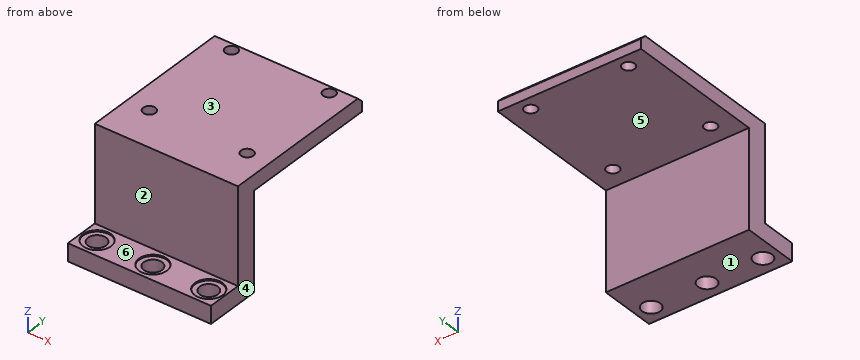
from build123d import *

# Parameters (mm, degrees)
EXTRUDE_1_DEPTH                 = 205
HOLE_WIZARD_M20_1_D             = 17.5
PATTERN_LINEAR_1_COUNT          = 2
PATTERN_LINEAR_1_PITCH          = 140
PATTERN_LINEAR_1_COUNT_DIR2     = 2
PATTERN_LINEAR_1_PITCH_DIR2     = 152
HOLE_WIZARD_M20_1_2_D           = 26
HOLE_WIZARD_M20_1_2_CBORE_D     = 40
HOLE_WIZARD_M20_1_2_CBORE_DEPTH = 2
PATTERN_LINEAR_2_COUNT          = 3
PATTERN_LINEAR_2_PITCH          = 80
CHAMFER_1_SIZE                  = 8


with BuildPart() as part:
    # 草图1 → 凸台-拉伸1 (new body)
    with BuildSketch(Plane(origin=(0, 0, 0), x_dir=(0, 0, -1), z_dir=(1, 0, 0))):
        Polygon((0, 0), (137, 0), (137, -50), (162, -50), (162, 30), (22, 30), (22, 230), (0, 230), align=None)
    extrude(amount=EXTRUDE_1_DEPTH)

    # Hole Wizard M20 _1 (through all)
    with Locations(Plane(origin=(32.5, 211, 0), x_dir=(1, 0, 0), z_dir=(0, 0, 1))):
        with Locations((0, 0)):
            hole_wizard_m20_1 = Hole(HOLE_WIZARD_M20_1_D / 2)

    # 阵列(线性)1: Hole Wizard M20 _1 2 × 2
    with Locations(*[(i * PATTERN_LINEAR_1_PITCH, -j * PATTERN_LINEAR_1_PITCH_DIR2, 0) for i in range(PATTERN_LINEAR_1_COUNT) for j in range(PATTERN_LINEAR_1_COUNT_DIR2) if (i, j) != (0, 0)]):
        add(hole_wizard_m20_1, mode=Mode.SUBTRACT)

    # Hole Wizard M20 _1 2 (through all)
    with Locations(Plane(origin=(22.5, -25, -137), x_dir=(0, 1, 0), z_dir=(0, 0, 1))):
        with Locations((0, 0)):
            hole_wizard_m20_1_2 = CounterBoreHole(HOLE_WIZARD_M20_1_2_D / 2, HOLE_WIZARD_M20_1_2_CBORE_D / 2, HOLE_WIZARD_M20_1_2_CBORE_DEPTH)

    # 阵列(线性)2: Hole Wizard M20 _1 2 ×3
    with Locations(*[(i * PATTERN_LINEAR_2_PITCH, 0, 0) for i in range(1, PATTERN_LINEAR_2_COUNT)]):
        add(hole_wizard_m20_1_2, mode=Mode.SUBTRACT)

    # 倒角1
    chamfer_1_edges = [part.edges().sort_by_distance(p)[0] for p in [
        (102.5, 230, 0),
    ]]
    chamfer(chamfer_1_edges, length=CHAMFER_1_SIZE)


solid = part.part
Source: CAD feature listing. Evaluate the final solid. Frame: model axes, mm. Face numbers are marked on the shaded views. A direction names the side the tool comes from. Round coordinates to 2 decimals unless told otherwise and drop trailing zeros. Loops run counter-clockwise (first coordinate to the right, second up) from the corner with the lowest first, then second, coordinate; pieces in that order, holes last. Notation, with made-up numbers: (-28, 5) - (-10, 5) arc R23 ccw to (-10, 41) - close; hole circle Ø3 at (-18, 46). An arc over 180 degrees is marked (long way). Write item = value, one per line. Start each with the question number.
Item 1: Section query C-C on x = 155. Output: boundary loops of the cut face in (y, z), plus the area to 3 significant figures.
Item 2: Section query B-B on x = 102.5. Output: boundary loops of the cut face in (y, z), plus the area to 3 significant figures.
Item 3: First-contact query: pin 1 Ø1.5 at (x, z) = (33.5, -42) entering from +Y; pin 2 Ø20 at (x, y) = (106.5, -26) entering from +Z; pin 3 Ø15.5 at (x, y) = (102.5, -25) entering from +Z (3 decimals); pin 4 Ø25 at (x, y) = (69.5, -33) entering from +Z. Flat tips, straight axial feed; report the tip coordinate or a pass-through.
Item 4: Reachability of the marked faces 4, 5 and 6 from +Z, -Z, +X, -X, +Y, -Y: full face, straight path, thin tool, end or side. Return the list, or none.
Item 5: Mould query, pull axis Z, two halves, no side actions, for the marked faces 1, 2 and 3. Classes: released by +Z, released by -Z, zero draft, split by the parting line, or undercut.
Item 6: Section query A-A on y = 211. Output: boundary loops of the cut face in (x, z), plus the area to 3 significant figures.
Item 7: Section query D-D on z = -104. Output: boundary loops of the cut face in (x, y), plus the area to 3 significant figures.
Item 8: Material intervals for line 1 (X direction, y = -25, z = -151); line 2 (X direction, y = -25, z = -137.6); line 3 (Y direction, x = 148.5, z = -101.5), sorted ascending.
Results list:
q1.outline = (-50, -162) - (30, -162) - (30, -22) - (230, -22) - (230, -8) - (222, 0) - (0, 0) - (0, -137) - (-50, -137) - close
q1.area = 10,500 mm²
q2.outline = (-50, -162) - (-38, -162) - (-38, -139) - (-45, -139) - (-45, -137) - (-50, -137) - close; (-12, -162) - (30, -162) - (30, -22) - (230, -22) - (230, -8) - (222, 0) - (0, 0) - (0, -137) - (-5, -137) - (-5, -139) - (-12, -139) - close
q2.area = 9,800 mm²
q3.pin_1 = 30
q3.pin_2 = -139
q3.pin_3 = through
q3.pin_4 = -137
q4.face_4 = +Z, -Z, +X, +Y, -Y
q4.face_5 = -Z, +X, -X, +Y
q4.face_6 = +Z, +X, -X, -Y
q5.face_1 = released by -Z
q5.face_2 = zero draft
q5.face_3 = released by +Z
q6.outline = (0, -22) - (23.75, -22) - (23.75, 0) - (0, 0) - close; (41.25, -22) - (163.75, -22) - (163.75, 0) - (41.25, 0) - close; (181.25, -22) - (205, -22) - (205, 0) - (181.25, 0) - close
q6.area = 3,740 mm²
q7.outline = (0, 0) - (205, 0) - (205, 30) - (0, 30) - close
q7.area = 6,150 mm²
q8.line_1 = 0 to 9.5, 35.5 to 89.5, 115.5 to 169.5, 195.5 to 205
q8.line_2 = 0 to 2.5, 42.5 to 82.5, 122.5 to 162.5, 202.5 to 205
q8.line_3 = 0 to 30
